from build123d import *

# Parameters (mm, degrees)
EXTRUDE_1_DEPTH          = 2
SKETCH_3_R               = 2
EXTRUDE_2_DEPTH          = 9
SKETCH_4_R               = 2
EXTRUDE_3_DEPTH          = 25
SKETCH_5_R               = 2.5
CUT_EXTRUDE_2_DEPTH      = 25
SKETCH_7_R               = 2.5
EXTRUDE_4_DEPTH          = 0.25
CUT_EXTRUDE_3_DEPTH      = 61.402419684
CUT_EXTRUDE_3_DEPTH_BACK = 10
SKETCH_8_W               = 14.774450984
SKETCH_8_H               = 5.235041687
SKETCH_8_W_2             = 21.085271114
SKETCH_8_H_2             = 10.942988806
SKETCH_9_W               = 2
SKETCH_9_H               = 10
EXTRUDE_5_DEPTH          = 54
EXTRUDE_START            = 13.5
SKETCH_10_R              = 1.5
EXTRUDE_6_DEPTH          = 2
FILLET_3_R               = 1
FILLET_3_OF_MIRROR_5_R   = 1


with BuildPart() as part:
    # 草圖1 → 填料-伸長1 (new body)
    with BuildSketch(Plane.XY):
        with BuildLine():
            Line((-48.07750061, -5), (51.758125458, -5))
            ThreePointArc((51.758125458, -5), (54.462035166, -3.299566191), (54.100731886, -0.125914857))
            Line((54.100731886, -0.125914857), (51.200975848, 3.49878019))
            ThreePointArc((51.200975848, 3.49878019), (49.810255532, 4.605212945), (48.07750061, 5))
            Line((48.07750061, 5), (-51.758125458, 5))
            ThreePointArc((-51.758125458, 5), (-54.462035166, 3.299566191), (-54.100731886, 0.125914857))
            Line((-54.100731886, 0.125914857), (-51.200975848, -3.49878019))
            ThreePointArc((-51.200975848, -3.49878019), (-49.810255532, -4.605212945), (-48.07750061, -5))
        make_face()
    extrude(amount=EXTRUDE_1_DEPTH)

    # 草圖3 → 填料-伸長2 (add)
    with BuildSketch(Plane.XY.offset(2)):
        with Locations((-51.758125458, 2)):
            Circle(SKETCH_3_R)
        with Locations((51.758125458, -2)):
            Circle(SKETCH_3_R)
    extrude(amount=EXTRUDE_2_DEPTH)

    # 草圖4 → 填料-伸長3 (add)
    with BuildSketch(Plane(origin=(0, 0, 0), x_dir=(-1, 0, 0), z_dir=(0, 0, -1))):
        with Locations(Location((-40, 2, 0), (0, 0, 180))):
            Circle(SKETCH_4_R)
        with Locations(Location((40, 2, 0), (0, 0, 180))):
            Circle(SKETCH_4_R)
    extrude(amount=EXTRUDE_3_DEPTH)

    # 草圖5 → 除料-伸長2 (cut)
    with BuildSketch(Plane(origin=(0, 0, 0), x_dir=(-1, 0, 0), z_dir=(0, 0, -1))):
        Circle(SKETCH_5_R)
    extrude(amount=-CUT_EXTRUDE_2_DEPTH, mode=Mode.SUBTRACT)

    # 草圖7 → 填料-伸長4 (add)
    with BuildSketch(Plane.XY.offset(2)):
        with Locations((51.758125458, -2)):
            Circle(SKETCH_7_R)
        with Locations((-51.758125458, 2)):
            Circle(SKETCH_7_R)
    extrude(amount=EXTRUDE_4_DEPTH)

    # 草圖8 → 除料-伸長3 (cut, two sides: drawn at the far end of the back side and taken through both)
    with BuildSketch(Plane(origin=(0, 0, 0), x_dir=(1, 0, 0), z_dir=(0, 1, 0)).offset(-CUT_EXTRUDE_3_DEPTH_BACK)):
        with Locations((49.50022751, -10.117520844)):
            Rectangle(SKETCH_8_W, SKETCH_8_H)
        with Locations((-50.795099296, -12.971494403)):
            Rectangle(SKETCH_8_W_2, SKETCH_8_H_2)
    extrude(amount=CUT_EXTRUDE_3_DEPTH + CUT_EXTRUDE_3_DEPTH_BACK, mode=Mode.SUBTRACT)

    # 鏡射1: part across plane


with BuildPart() as part_1:
    add(part.part)
    add(part.part.mirror(Plane(origin=(-40, 2, -25), x_dir=(1, 0, 0), z_dir=(0, 0, 1))))

    # 草圖9 → 填料-伸長5 (add)
    with BuildSketch(Plane.XY.offset(2)):
        with Locations((-24, 0)):
            Rectangle(SKETCH_9_W, SKETCH_9_H)
    extrude(amount=-EXTRUDE_5_DEPTH)

    # 草圖10 → 填料-伸長6 (add)
    with BuildSketch(Plane(origin=(0, 0, -25), x_dir=(-1, 0, 0), z_dir=(0, 0, -1)).offset(EXTRUDE_START)):
        with BuildLine():
            Line((23, 2.5), (20.5, 2.5))
            ThreePointArc((20.5, 2.5), (18, 0), (20.5, -2.5))
            Line((20.5, -2.5), (23, -2.5))
            Line((23, -2.5), (23, 2.5))
        make_face()
        with Locations((20.5, 0)):
            Circle(SKETCH_10_R, mode=Mode.SUBTRACT)
    extrude_6 = extrude(amount=EXTRUDE_6_DEPTH)

    # 圓角3
    fillet_3_edges = [part_1.edges().sort_by_distance(p)[0] for p in [
        (-23, 0, -40.5),
        (-23, 0, -38.5),
        (-23, -2.5, -39.5),
        (-23, 2.5, -39.5),
    ]]
    fillet(fillet_3_edges, radius=FILLET_3_R - 0.0001)  # a hair under: the kernel refuses the full size

    # 鏡射5: 填料-伸長6 across plane
    add(extrude_6.mirror(Plane(origin=(0, 0, -25), x_dir=(1, 0, 0), z_dir=(0, 0, -1))))

    # 圓角3 of 鏡射5
    fillet_3_of_mirror_5_edges = [part_1.edges().sort_by_distance(p)[0] for p in [
        (-23, 0, -9.5),
        (-23, 0, -11.5),
        (-23, -2.5, -10.5),
        (-23, 2.5, -10.5),
    ]]
    fillet(fillet_3_of_mirror_5_edges, radius=FILLET_3_OF_MIRROR_5_R - 0.0001)  # a hair under: the kernel refuses the full size


solid = part_1.part
CAD build for the part. Positions are in the model's coordinates, mm. A direction names the side the tool comes from. Give positions to 0.01 mm unless a question says otherwise; leave off trailing zeros. Order: outer loops, then holes, each group sorted by start corner. A loop starts at its lowest first (then second) coordinate and runs counter-clockwise, first axis right, second up. Notation, with made-up numbers: (-24, 83) -> (1, 83) arc R5 ccw to (1, 89) -> close; hole circle Ø7 at (48.5, -39). An arc over 180 degrees is marked (long way). Return JSON: item names as keys, results as strings.
Q1. Saw through at A-A (x = -30). Write the cut outline in (y, z), then the cut area to 3 significant figures.
Working result:
{"outline": "(-5, -52) -> (5, -52) -> (5, -50) -> (-5, -50) -> close; (-5, 0) -> (5, 0) -> (5, 2) -> (-5, 2) -> close", "area": "40.0 mm²"}
Q2. Drill centre lines: line 1 (Z direction, x = 47.5, y = 1.25); line 2 (X direction, y = 1.5, z = -29); line 3 (Y direction, x = 0, z = -51). Where is each one in solid material? Low to high.
Working result:
{"line 1": "-52 to -50, 0 to 2", "line 2": "-41.94 to -38.06, -25 to -23, 38.06 to 41.94", "line 3": "-5 to -2.5, 2.5 to 5"}
Q3. Which spindle directions (+Z, -Z, +X, -X, +Y, -Y) get a long thin tool onto all of the face, cutting with end or side? Do faces 4 (the face through (-49.911, 1.234, -54.838)), 5 (the face through (-18, 0, -11)), 6 (the face through (-19, -1, -38.5)), 7 (the face through (49.76, -1.91, 4.84)). Say none if no direction does.
Working result:
{"face 4": "-Z", "face 5": "none", "face 6": "+Y, -Y", "face 7": "+Z"}
Q4. Flat gauge pins, fed straight in: pin 1 (12 mm diameter, centred on x = -37, z = -48, fed in from -Y); pin 2 (1.5 mm diameter, centred on y = 0.5, z = -43.5, fed in from +X); pin 3 (3 mm diameter, centred on y = -0.5, z = -43.5, fed in from -X); pin 4 (0.5 mm diameter, centred on x = -21, z = -10, fed in from +Y). Where does each tip first touch, or does it go through?
Working result:
{"pin 1": "y = -5", "pin 2": "x = 41.85", "pin 3": "x = -41.73", "pin 4": "y = 2.5"}
Q5. Mould opens along Z. For faces 1 (the face through (-52.67, -1.66, 0.99)), 2 (the face through (-1, -3, 2)), 3 (the face through (-40, -1, 0)) say: pulls with the +Z half, pulls with the -Z half, needs draft (parallel to the pull), parting line crosses it, or undercut.
Working result:
{"face 1": "needs draft", "face 2": "pulls with the +Z half", "face 3": "undercut"}
Q6. Saw through at C-C (z = -36). Write the cut outline in (x, y), then the cut area to 3 significant figures.
Working result:
{"outline": "circle Ø4 at (-40, 2); (-25, -5) -> (-23, -5) -> (-23, 5) -> (-25, 5) -> close; circle Ø4 at (40, 2)", "area": "45.1 mm²"}
Q7. Saw through at B-B (x = 0). Write the cut outline in (y, z), then the cut area to 3 significant figures.
Working result:
{"outline": "(-5, -52) -> (-2.5, -52) -> (-2.5, -50) -> (-5, -50) -> close; (-5, 0) -> (-2.5, 0) -> (-2.5, 2) -> (-5, 2) -> close; (2.5, -52) -> (5, -52) -> (5, -50) -> (2.5, -50) -> close; (2.5, 0) -> (5, 0) -> (5, 2) -> (2.5, 2) -> close", "area": "20.0 mm²"}
Q8. Saw through at D-D (x = 40). Write the cut outline in (y, z), then the cut area to 3 significant figures.
Working result:
{"outline": "(-5, -52) -> (5, -52) -> (5, -50) -> (4, -50) -> (4, 0) -> (5, 0) -> (5, 2) -> (-5, 2) -> (-5, 0) -> (0, 0) -> (0, -50) -> (-5, -50) -> close", "area": "240 mm²"}
